Source: three-view drawing plus pictorial views. Frame: mm from the lowest corner of the part. A direction names the side the tool comes from. Coordinates: 2 decimals unless noted, no trailing zeros. Write each loop counter-clockwise with the first axis right and the second up, starting at its lowest first coordinate (ties: lowest second). Pieces come first, ordered by that corner, then holes. Notation, with made-up numbers: (71, 82.5) - (89, 82.5) arc R26 ccw to (89, 97.5) - close; hole circle Ø9 at (-36.5, 29). An arc over 180 degrees is marked (long way). One line per item, written item: value.
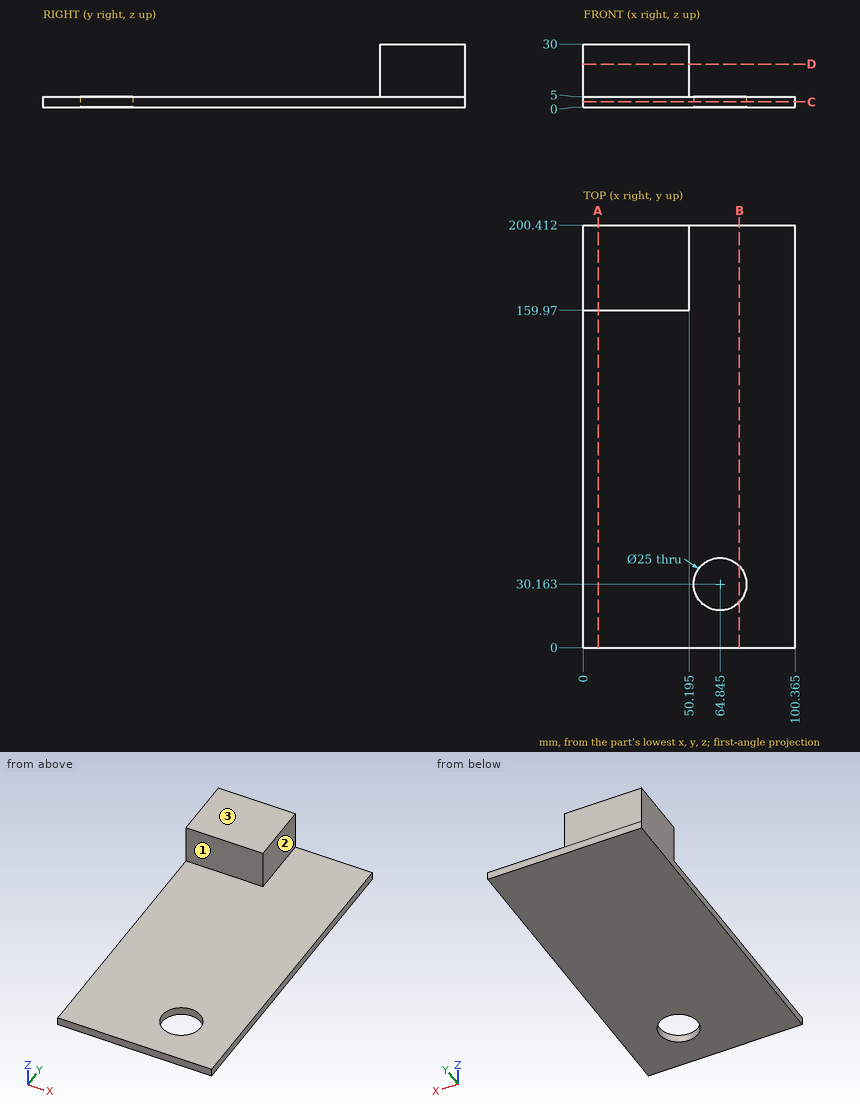
1) Section query C-C on z = 2.5. Output: boundary loops of the cut face in (x, y) (1 decimal).
Values found:
outline: (0, 0) - (100.4, 0) - (100.4, 200.4) - (0, 200.4) - close; hole circle Ø25 at (64.8, 30.2)
2) Section query B-B on x = 74. Output: boundary loops of the cut face in (y, z), then the cut area to 3 significant figures.
Values found:
outline: (0, 0) - (21.65, 0) - (21.65, 5) - (0, 5) - close; (38.67, 0) - (200.41, 0) - (200.41, 5) - (38.67, 5) - close
area: 917 mm2
3) Section query A-A on x = 7. Output: boundary loops of the cut face in (y, z).
Values found:
outline: (0, 0) - (200.41, 0) - (200.41, 30) - (159.97, 30) - (159.97, 5) - (0, 5) - close
4) Material intervals for line 1 (Z direction, x = 42, y = 29.5); line 2 (X direction, y = 172, z = 9.5) (1 decimal); line 3 (Y direction, x = 29.5, z = 10), sorted ascending.
Values found:
line 1: 0 to 5
line 2: 0 to 50.2
line 3: 159.97 to 200.41
5) Section query D-D on z = 20.5. Output: boundary loops of the cut face in (x, y) (1 decimal), then the cut area to 3 significant figures.
Values found:
outline: (0, 160) - (50.2, 160) - (50.2, 200.4) - (0, 200.4) - close
area: 2,030 mm2
6) Reachability of the marked faces 1, 2 and 3 from +Z, -Z, +X, -X, +Y, -Y: full face, straight path, thin tool, end or side. Return the list, or none.
Values found:
face 1: +Z, +X, -X, -Y
face 2: +Z, +X, +Y, -Y
face 3: +Z, +X, -X, +Y, -Y
7) Contact query for flat-ended pins moving along their axis: P1, Ø5, axis at x = 60.5, y = 152, coming from the +Z side; P2, Ø3, axis at x = 21.5, z = 14.5, coming from the -Y side. Output: stop coordinate, or through.
Values found:
P1: z = 5
P2: y = 159.97
